Part model, mm, in its own coordinate system. A direction names the side the tool comes from. Round coordinates to 2 decimals unless told otherwise and drop trailing zeros. Loops run counter-clockwise (first coordinate to the right, second up) from the corner with the lowest first, then second, coordinate; pieces in that order, holes last. Notation, with made-up numbers: M 20.5,-8.75 L 26.5,-8.75 A19 cw 26.5,21.25 Z; hole C 33,25 d5. An arc over 180 degrees is marked long. Put each result on its own line as item: value. Start each with the question number.
```python
from build123d import *

# Parameters (mm, degrees)
F1_DEPTH = 6.35
F2_R     = 2
F3_DEPTH = 22.5
F4_R     = 5
F5_R     = 1.75
F6_DEPTH = 28.001


# Not quite as in the source:
# - a feature names something its author has since deleted; it is built from what else it names


with BuildPart() as f1:
    # F0 (on Front) → F1 (new body)
    with BuildSketch(Plane.XZ):
        with BuildLine():
            ThreePointArc((0, -3.96875), (-3.96875, 0), (0, 3.96875))
            Line((0, 3.96875), (0, 9.525))
            Line((0, 9.525), (-8, 9.525))
            Line((-8, 9.525), (-8, 3.1353827518))
            ThreePointArc((-8, 3.1353827518), (-6.0846195952, 2.0607189279), (-5.325, 0))
            ThreePointArc((-5.325, 0), (-10.5607189279, -2.4153804048), (-9, 3.1353827518))
            Line((-9, 3.1353827518), (-9, 9.525))
            Line((-9, 9.525), (-14, 9.525))
            Line((-14, 9.525), (-14, -6.35))
            Line((-14, -6.35), (0, -6.35))
            Line((0, -6.35), (0, -3.96875))
        make_face()
        with BuildLine():
            ThreePointArc((0, 3.96875), (2.8063300378, 2.8063300378), (3.96875, 0))
            ThreePointArc((3.96875, 0), (2.8063300378, -2.8063300378), (0, -3.96875))
            Line((0, -3.96875), (0, -6.35))
            Line((0, -6.35), (14, -6.35))
            Line((14, -6.35), (14, 9.525))
            Line((14, 9.525), (9, 9.525))
            Line((9, 9.525), (9, 3.1353827518))
            ThreePointArc((9, 3.1353827518), (10.9153804048, 2.0607189279), (11.675, 0))
            ThreePointArc((11.675, 0), (6.4392810721, -2.4153804048), (8, 3.1353827518))
            Line((8, 3.1353827518), (8, 9.525))
            Line((8, 9.525), (0, 9.525))
            Line((0, 9.525), (0, 3.96875))
        make_face()
    extrude(amount=F1_DEPTH)

    # F2 (on face) → F3 (cut)
    with BuildSketch(Plane.YZ.offset(14)):
        with Locations((-3.175, 6.35)):
            Circle(F2_R)
    extrude(amount=-F3_DEPTH, mode=Mode.SUBTRACT)

    # F4
    f4_edges = [f1.edges().sort_by_distance(p)[0] for p in [
        (14, -3.175, -6.35),
        (-14, -3.175, -6.35),
    ]]
    fillet(f4_edges, radius=F4_R)

    # F5 (on face) → F6 (cut, through all)
    with BuildSketch(Plane(origin=(-14, 0, 0), x_dir=(0, -1, 0), z_dir=(-1, 0, 0))):
        with Locations((3.175, 6.35)):
            Circle(F5_R)
    extrude(amount=-F6_DEPTH, mode=Mode.SUBTRACT)


solid = f1.part
```
1. Which spindle directions (+Z, -Z, +X, -X, +Y, -Y) get a long thin tool onto all of the face, cutting with end or side? Do faces 4 (the flat face through (9, -1, 6)), 5 (the cylindrical face through (11.535, -3.609, 4.398)), 6 (the flat face through (12, -3, 9.525)). Say none if no direction does.
2. Wall check: L1, parallel to X at y = -0.75, z = 5.5; L2, parallel to X at y = -4, z = -1.75; L3, parallel to Z at x = 11.25, y = -2 (3 decimals). Give the ranges that are in metal, low to high.
3. Mould opens along Y. For faces 1 (the flat face through (0, -6.35, 5)), 2 (the flat face through (0, -3, -6.35)), 3 (the cylindrical face through (0.112, -3.609, 4.398)) say: released by +Y, released by -Y, zero draft, split by the parting line, or undercut.
4. Cut at A-A, the plane z = 6.35. Give the cut face in (x, y) (3 decimals), and give its area (3 significant figures).
5. Cut at C-C, the plane x = 6.5. Give the cut face in (y, z) (3 decimals).
6. Cut at B-B, the plane y = -1.75. Give the number of separate pieces and of enclosed holes in the cut face, and give its area (3 significant figures).
7. Cut at D-D, the plane z = 1. Give the cut face in (x, y).
Results list:
1. face 4: +Z, +Y, -Y
1. face 5: +X
1. face 6: +Z, +X, -X, +Y, -Y
2. L1: x = -14 to -9, -8 to 8, 9 to 14
2. L2: x = -13.98 to -11.15, -5.85 to -3.56, 3.56 to 5.85, 11.15 to 13.98
2. L3: z = -5.815 to -1.587, 1.587 to 4.732, 7.968 to 9.525
3. face 1: released by -Y
3. face 2: zero draft
3. face 3: undercut
4. outline: M -14,-6.35 L -9,-6.35 L -9,-4.925 L -14,-4.925 Z; M -14,-1.425 L -9,-1.425 L -9,0 L -14,0 Z; M -8,-6.35 L 8,-6.35 L 8,-5.175 L -8,-5.175 Z; M -8,-1.175 L 8,-1.175 L 8,0 L -8,0 Z; M 9,-6.35 L 14,-6.35 L 14,-5.175 L 9,-5.175 Z; M 9,-1.175 L 14,-1.175 L 14,0 L 9,0 Z
4. area: 63.6 mm^2
5. outline: M -6.35,-6.35 L 0,-6.35 L 0,-2.466 L -6.35,-2.466 Z; M -6.35,2.466 L 0,2.466 L 0,9.525 L -6.35,9.525 Z; hole C -3.175,6.35 d4
6. separate pieces: 4
6. enclosed holes: 1
6. area: 239 mm^2
7. outline: M -14,-6.35 L -11.51,-6.35 L -11.51,0 L -14,0 Z; M -5.49,-6.35 L -3.84,-6.35 L -3.84,0 L -5.49,0 Z; M 3.84,-6.35 L 5.49,-6.35 L 5.49,0 L 3.84,0 Z; M 11.51,-6.35 L 14,-6.35 L 14,0 L 11.51,0 Z
